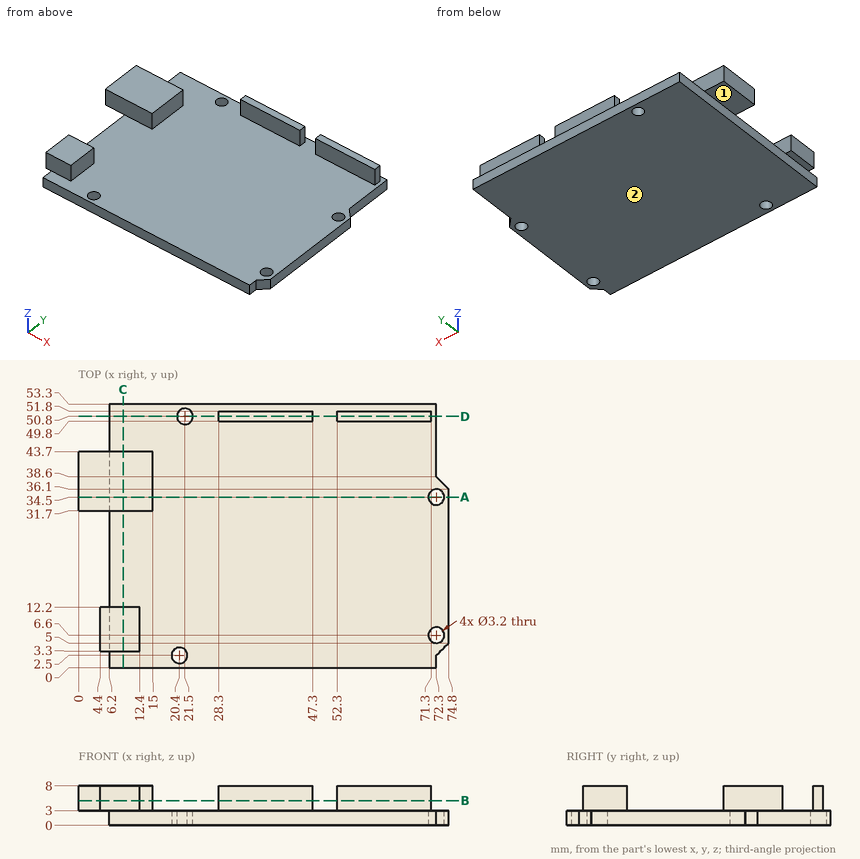
Print and shaded views of the part. All mm, measured from the part's lowest x, y and z. A direction names the side the tool comes from. Give positions to 0.01 mm unless a question says otherwise; leave off trailing zeros. Write each loop counter-clockwise with the first axis right and the second up, starting at its lowest first coordinate (ties: lowest second). Pieces come first, ordered by that corner, then holes. Notation, with made-up numbers: M 67,47 L 109,47 A32 ccw 109,80 Z; hole C 37.5,89.5 d9. An arc over 180 degrees is marked long. Use a Markdown table: item, result.
1) Cut at C-C (x = 9). List the corners of the cut face in (y, z), and give its area (3 significant figures).
Responses:
| item | result |
|---|---|
| outline | M 0,0 L 53.3,0 L 53.3,3 L 43.7,3 L 43.7,8 L 31.7,8 L 31.7,3 L 12.2,3 L 12.2,8 L 3.3,8 L 3.3,3 L 0,3 Z |
| area | 264 mm2 |
2) Cut at D-D (y = 50.8). List the corners of the cut face in (x, z).
Responses:
| item | result |
|---|---|
| outline | M 6.2,0 L 19.9,0 L 19.9,3 L 6.2,3 Z; M 23.1,0 L 72.3,0 L 72.3,3 L 71.3,3 L 71.3,8 L 52.3,8 L 52.3,3 L 47.3,3 L 47.3,8 L 28.3,8 L 28.3,3 L 23.1,3 Z |
3) Cut at A-A (y = 34.5). List the corners of the cut face in (x, z), and give its area (3 significant figures).
Responses:
| item | result |
|---|---|
| outline | M 0,3 L 6.2,3 L 6.2,0 L 70.7,0 L 70.7,3 L 15,3 L 15,8 L 0,8 Z; M 73.9,0 L 74.8,0 L 74.8,3 L 73.9,3 Z |
| area | 271 mm2 |
4) Pin check, flat tips, straight feed: pin 1 (6 mm diameter, centred on x = 66, y = 13, fed in from +Z); pin 2 (1 mm diameter, centred on y = 51, z = 5, fed in from +X); pin 3 (1.5 mm diameter, centred on y = 11.5, z = 5, fed in from +X). Stop position of each tip, or through.
Responses:
| item | result |
|---|---|
| pin 1 | stops at z = 3 |
| pin 2 | stops at x = 71.3 |
| pin 3 | stops at x = 12.4 |
5) Tool access for the marked faces 1 and 2: list every direction of +Z, -Z, +X, -X, +Y, -Y with a clear straight run to the whole face (end or side of a thin tool).
Responses:
| item | result |
|---|---|
| face 1 | -Z, -X, +Y, -Y |
| face 2 | -Z, +X, -X, +Y, -Y |
6) Cut at B-B (z = 5). List the corners of the cut face in (x, y).
Responses:
| item | result |
|---|---|
| outline | M 0,31.7 L 15,31.7 L 15,43.7 L 0,43.7 Z; M 4.4,3.3 L 12.4,3.3 L 12.4,12.2 L 4.4,12.2 Z; M 28.3,49.8 L 47.3,49.8 L 47.3,51.8 L 28.3,51.8 Z; M 52.3,49.8 L 71.3,49.8 L 71.3,51.8 L 52.3,51.8 Z |
7) Drill centre lines: line 1 (Y direction, x = 20.4, z = 1.65); line 2 (Y direction, x = 21.5, z = 2.2); line 3 (Y direction, x = 5.5, z = 6.25). Where is each one in solid material? Low to high. Write a range as from..to.
Responses:
| item | result |
|---|---|
| line 1 | y = 0..0.9, 4.1..49.64, 51.96..53.3 |
| line 2 | y = 0..1.34, 3.66..49.2, 52.4..53.3 |
| line 3 | y = 3.3..12.2, 31.7..43.7 |
